Can you work these out from the drawing? Everything is in mm from the part's minimum corner. Round coordinates to 2 decimals unless told otherwise and drop trailing zeros. Order: outer loops, then holes, each group sorted by start corner. A loop starts at its lowest first (then second) coordinate and runs counter-clockwise, first axis right, second up. Notation, with made-up numbers: M -7.75,57.25 L 30.25,57.25 A29 ccw 30.25,80.25 Z; hole C -36,24 d7. An arc over 180 degrees is marked long. Answer as CSV lines item,"result". Start each with the question number.
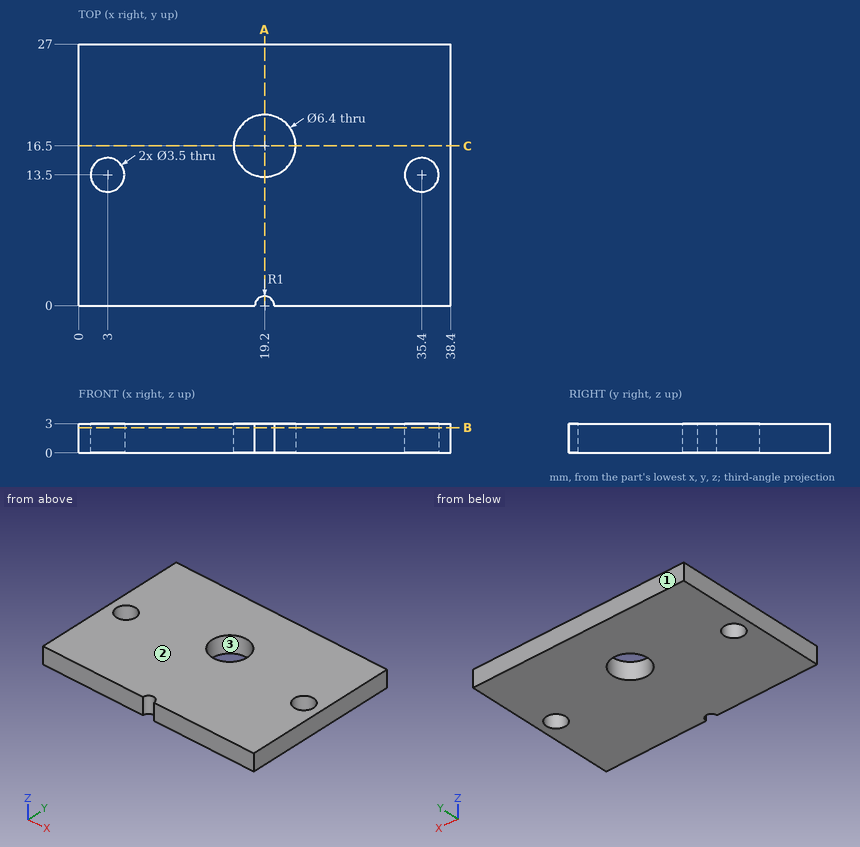
(1) I want a section at B-B on z = 2.6. Write out the boundary of the cut face in (x, y), and give its area (3 significant figures).
(2) I want a section at C-C on y = 16.5. Write out the boundary of the cut face in (x, z).
(3) If I drill on line 1 along Y through (x, z) = (3, 2.3); line 2 along Y through (x, z) = (19.2, 0.95); line 3 along X through (y, z) = (16, 1.95), over which ranges is the centre line in solid material (lowest first)?
(4) I want a section at A-A on x = 19.2. Write out the boundary of the cut face in (y, z).
(5) If we mould it in two halves opening along Y, with no side actions, what happens to the marked faces 1, 2 and 3? For each: +Y half, -Y half, draft (parallel to the pull), parting line (faces both ways), or undercut.
(6) I'm going to push flat-ended pins straight in: P1, Ø4.5, axis at x = 35.4, y = 13.5, coming from the -Z side; P2, Ø6, axis at x = 19.2, y = 16.5, coming from the +Z side. Where does each tip first touch, or does it pass through?
From the geometry:
1,outline,"M 0,0 L 18.2,0 A1 cw 20.2,0 L 38.4,0 L 38.4,27 L 0,27 Z; hole C 3,13.5 d3.5; hole C 19.2,16.5 d6.4; hole C 35.4,13.5 d3.5"
1,area,"984 mm²"
2,outline,"M 0,0 L 16,0 L 16,3 L 0,3 Z; M 22.4,0 L 38.4,0 L 38.4,3 L 22.4,3 Z"
3,line 1,"0 to 11.75, 15.25 to 27"
3,line 2,"1 to 13.3, 19.7 to 27"
3,line 3,"0 to 16.04, 22.36 to 38.4"
4,outline,"M 1,0 L 13.3,0 L 13.3,3 L 1,3 Z; M 19.7,0 L 27,0 L 27,3 L 19.7,3 Z"
5,face 1,"+Y half"
5,face 2,"draft"
5,face 3,"undercut"
6,P1,"z = 0"
6,P2,"through"
